from build123d import *

# Parameters (mm, degrees)
SKETCH_1_W      = 117
SKETCH_1_H      = 87
SKETCH_1_W_2    = 110
SKETCH_1_H_2    = 80
EXTRUDE_1_DEPTH = 3
SKETCH_2_W      = 117
SKETCH_2_H      = 87
SKETCH_2_W_2    = 109.279406394
SKETCH_2_H_2    = 78.35290245
EXTRUDE_2_DEPTH = 15


with BuildPart() as part:
    # 草图1 → 凸台-拉伸1 (new body)
    # profile 1 of 2: a face of its own
    with BuildSketch(Plane.XY):
        with Locations((58.5, -43.5)):
            Rectangle(SKETCH_1_W, SKETCH_1_H)
        with Locations((58.5, -43.5)):
            Rectangle(SKETCH_1_W_2, SKETCH_1_H_2, mode=Mode.SUBTRACT)
    # profile 2 of 2: a face of its own
    with BuildSketch(Plane.XY):
        with Locations((58.5, -43.5)):
            Rectangle(SKETCH_1_W_2, SKETCH_1_H_2)
    extrude(amount=EXTRUDE_1_DEPTH)

    # 草图2 → 凸台-拉伸2 (add)
    with BuildSketch(Plane.XY.offset(3)):
        with Locations((58.5, -43.5)):
            Rectangle(SKETCH_2_W, SKETCH_2_H)
        with Locations((58.139703197, -42.676451225)):
            Rectangle(SKETCH_2_W_2, SKETCH_2_H_2, mode=Mode.SUBTRACT)
    extrude(amount=EXTRUDE_2_DEPTH)


solid = part.part
CAD build for the part. Positions are in the model's coordinates, mm. A direction names the side the tool comes from. Give positions to 0.01 mm unless a question says otherwise; leave off trailing zeros. Order: outer loops, then holes, each group sorted by start corner. A loop starts at its lowest first (then second) coordinate and runs counter-clockwise, first axis right, second up. Notation, with made-up numbers: (72.25, -8.5) - (126.25, -8.5) arc R29 cw to (126.25, 12.5) - close; hole circle Ø7 at (-3, 41.25). An arc over 180 degrees is marked (long way). Answer in a Markdown table with one row per item.
1. Saw through at C-C, the plane x = 44. Give the cut face in (y, z), plus the area to 3 significant figures.
Data:
| item | result |
|---|---|
| outline | (-87, 0) - (0, 0) - (0, 18) - (-3.5, 18) - (-3.5, 3) - (-81.85, 3) - (-81.85, 18) - (-87, 18) - close |
| area | 391 mm² |
2. Saw through at A-A, the plane z = 8.5. Give the cut face in (x, y), plus the area to 3 significant figures.
Data:
| item | result |
|---|---|
| outline | (0, -87) - (117, -87) - (117, 0) - (0, 0) - close; hole (3.5, -81.85) - (112.78, -81.85) - (112.78, -3.5) - (3.5, -3.5) - close |
| area | 1,620 mm² |
3. Tool access for faces 1 (the flat face through (112.779, -43, 10)), 2 (the flat face through (0, -44, 9)): list every direction of +Z, -Z, +X, -X, +Y, -Y with a clear straight run to the whole face (end or side of a thin tool).
Data:
| item | result |
|---|---|
| face 1 | +Z |
| face 2 | +Z, -Z, -X, +Y, -Y |
4. Flat gauge pin, fed straight in: pin 1 (12 mm diameter, centred on x = 19.5, y = -68.5, fed in from +Z). Where does the tip first touch, or does it go through?
Data:
| item | result |
|---|---|
| pin 1 | stops at z = 3 |
5. Saw through at B-B, the plane y = -79. Give the cut face in (x, z).
Data:
| item | result |
|---|---|
| outline | (0, 0) - (117, 0) - (117, 18) - (112.78, 18) - (112.78, 3) - (3.5, 3) - (3.5, 18) - (0, 18) - close |
6. Pull direction X, two halves, no side cores. Call faces 3 (the flat face through (117, -44, 9)), 4 (the flat face through (3.5, -43, 10)), 5 (the flat face through (58, -43, 0)): pulls with the +X half, pulls with the -X half, needs draft (parallel to the pull), parting line crosses it, or undercut.
Data:
| item | result |
|---|---|
| face 3 | pulls with the +X half |
| face 4 | undercut |
| face 5 | needs draft |
7. Probe probe 1 along X at (y, z) = (-18.5, 12.75); probe 2 along Y at (x, z) = (45, 9.25); probe 3 along Z at (x, y) = (51, -48.5). List the from-to ranges inside material, lowest first. Write a range as [from, to].
Data:
| item | result |
|---|---|
| probe 1 | x = [0, 3.5], [112.78, 117] |
| probe 2 | y = [-87, -81.85], [-3.5, 0] |
| probe 3 | z = [0, 3] |
